Design review of the part built by this model. Coordinates are the model's own, in mm. A direction names the side the tool comes from. Coordinates: 2 decimals unless noted, no trailing zeros. Order: outer loops, then holes, each group sorted by start corner. A loop starts at its lowest first (then second) coordinate and runs counter-clockwise, first axis right, second up. Notation, with made-up numbers: M -19,51 L 19,51 A30 cw 19,77 Z; hole C 87,49.25 d8. An arc over 180 degrees is marked long. Answer as a JSON object with one key per item and string values.
from build123d import *

# Parameters (mm, degrees)
SKETCH001_R          = 2.5
PAD_DEPTH            = 7.5
PAD_DEPTH_BACK       = 1.5
SKETCH_R             = 1.75
SKETCH_R_2           = 2.5
PAD001_DEPTH         = 6
SKETCH003_W          = 20
SKETCH003_H          = 3
POCKET_DEPTH         = 100
POCKET_DEPTH_BACK    = -100
FILLET_R             = 5
FILLET001_R          = 2
FILLET002_R          = 1
SKETCH004_R          = 4.25
POCKET001_DEPTH      = 2
POCKET001_DEPTH_BACK = -2
SKETCH005_R          = 5.5
POCKET002_DEPTH      = 5
SKETCH006_R          = 2.25
POCKET003_DEPTH      = 4


with BuildPart() as part:
    # Sketch001 → Pad (new body, two sides)
    with BuildSketch(Plane.XY) as pad_sk:
        Polygon((74, -6), (74, 0), (0, 0), (0, -6), (6.75, -6), (6.75, -20.25), (17.25, -20.25), (17.25, -6), (46.75, -6), (46.75, -20.25), (57.25, -20.25), (57.25, -6), align=None)
        with Locations((12, -15)):
            Circle(SKETCH001_R, mode=Mode.SUBTRACT)
        with Locations((52, -15)):
            Circle(SKETCH001_R, mode=Mode.SUBTRACT)
    extrude(amount=PAD_DEPTH)
    extrude(pad_sk.sketch, amount=-PAD_DEPTH_BACK)

    # Sketch → Pad001 (join)
    with BuildSketch(Plane.XZ):
        with BuildLine():
            ThreePointArc((37.87, 12.75), (34.37, 16.25), (30.87, 12.75))
            Line((30.87, 12.75), (30.87, 4.75))
            ThreePointArc((30.87, 4.75), (34.37, 1.25), (37.87, 4.75))
            Line((37.87, 12.75), (37.87, 4.75))
        make_face()
        with Locations((34.37, 12.75)):
            Circle(SKETCH_R, mode=Mode.SUBTRACT)
        with BuildLine():
            ThreePointArc((52.8, 12.75), (48.3, 17.25), (43.8, 12.75))
            Line((43.8, 12.75), (43.8, 4.75))
            ThreePointArc((43.8, 4.75), (48.3, 0.25), (52.8, 4.75))
            Line((52.8, 12.75), (52.8, 4.75))
        make_face()
        with Locations((48.3, 12.75)):
            Circle(SKETCH_R_2, mode=Mode.SUBTRACT)
        with BuildLine():
            ThreePointArc((69.87, 12.75), (66.37, 16.25), (62.87, 12.75))
            Line((62.87, 12.75), (62.87, 4.75))
            ThreePointArc((62.87, 4.75), (66.37, 1.25), (69.87, 4.75))
            Line((69.87, 12.75), (69.87, 4.75))
        make_face()
        with Locations((66.37, 12.75)):
            Circle(SKETCH_R, mode=Mode.SUBTRACT)
    extrude(amount=PAD001_DEPTH)

    # Sketch003 → Pocket (cut, two sides)
    with BuildSketch(Plane.YZ) as pocket_sk:
        with Locations((-12.2, 3)):
            Rectangle(SKETCH003_W, SKETCH003_H)
    extrude(amount=-POCKET_DEPTH, mode=Mode.SUBTRACT)
    extrude(pocket_sk.sketch, amount=-POCKET_DEPTH_BACK, mode=Mode.SUBTRACT)

    # Fillet
    fillet_edges = [part.edges().sort_by_distance(p)[0] for p in [
        (46.75, -20.25, 0),
        (46.75, -20.25, 6),
        (57.25, -20.25, 6),
        (57.25, -20.25, 0),
        (17.25, -20.25, 0),
        (17.25, -20.25, 6),
        (6.75, -20.25, 6),
        (6.75, -20.25, 0),
    ]]
    fillet(fillet_edges, radius=FILLET_R)

    # Fillet001
    fillet001_edges = [part.edges().sort_by_distance(p)[0] for p in [
        (74, 0, 3),
        (0, 0, 3),
    ]]
    fillet(fillet001_edges, radius=FILLET001_R)

    # Fillet002
    fillet002_edges = [part.edges().sort_by_distance(p)[0] for p in [
        (49.775, -6, 7.5),
        (52.8, -3, 7.5),
        (46.75, -6, 6),
        (57.25, -6, 6),
        (62.87, -3, 7.5),
        (69.87, -3, 7.5),
        (57.25, -6, 0),
        (46.75, -6, 0),
        (6.75, -6, 6),
        (6.75, -6, 0),
        (43.8, -3, 7.5),
        (30.87, -3, 7.5),
        (37.87, -3, 7.5),
        (17.25, -6, 6),
        (17.25, -6, 0),
    ]]
    fillet(fillet002_edges, radius=FILLET002_R)

    # Sketch004 → Pocket001 (cut, two sides)
    with BuildSketch(Plane.XY) as pocket001_sk:
        with Locations((12, -15)):
            Circle(SKETCH004_R)
        with Locations((52, -15)):
            Circle(SKETCH004_R)
    extrude(amount=-POCKET001_DEPTH, mode=Mode.SUBTRACT)
    extrude(pocket001_sk.sketch, amount=-POCKET001_DEPTH_BACK, mode=Mode.SUBTRACT)

    # Sketch005 → Pocket002 (cut)
    with BuildSketch(Plane.XY.offset(6.9)):
        with Locations((12, -15)):
            Circle(SKETCH005_R)
        with Locations((52, -15)):
            Circle(SKETCH005_R)
    extrude(amount=POCKET002_DEPTH, mode=Mode.SUBTRACT)

    # Sketch006 → Pocket003 (cut)
    with BuildSketch(Plane.XZ):
        with Locations((34.37, 12.75)):
            Circle(SKETCH006_R)
        with Locations((66.37, 12.75)):
            Circle(SKETCH006_R)
    extrude(amount=POCKET003_DEPTH, mode=Mode.SUBTRACT)


solid = part.part
1) Tool access review of faces 4 (the cylindrical face through (52.1, -9.5, 7.2)), 5 (the flat face through (46.75, -11, 0)), 6 (the cylindrical face through (48.63, -17.59, 0.02)): name each direction out of +Z, -Z, +X, -X, +Y, -Y from which nothing blocks a thin tool from reaching the whole face with its end or side.
Taken from the geometry:
{"face 4": "+Z, -Y", "face 5": "+Z, -Z, -Y", "face 6": "-Z"}
2) Mouldability with a two-part tool opening along Z and no side actions: class faces 1 (the flat face through (36, -3, -1.5)), 2 (the flat face through (36, -2.2, 3)), 3 (the flat face through (57.25, -11, 0)) as released by +Z, released by -Z, zero draft, split by the parting line, or undercut.
Taken from the geometry:
{"face 1": "released by -Z", "face 2": "undercut", "face 3": "zero draft"}
3) Add section C-C (x = 8.5). State the section outline as (y, z) points.
Taken from the geometry:
{"outline": "M -19.05,-1.5 L -17.41,-1.5 L -17.41,1.5 L -19.05,1.5 Z; M -19.05,4.5 L -2.2,4.5 L -2.2,1.5 L -12.59,1.5 L -12.59,-1.5 L 0,-1.5 L 0,7.5 L -10.76,7.5 L -10.76,6.9 L -19.05,6.9 Z"}
4) Add section A-A (x = 34.37). State the section outline as (y, z) points.
Taken from the geometry:
{"outline": "M -6,-1.5 L 0,-1.5 L 0,10.5 L -4,10.5 L -4,11 L -6,11 L -6,4.5 L -2.2,4.5 L -2.2,1.5 L -6,1.5 Z; M -6,14.5 L -4,14.5 L -4,15 L 0,15 L 0,16.25 L -6,16.25 Z"}
5) Insertion check: pin 1 Ø2 at (y, z) = (-4, 10.5) entering from +X; pin 2 Ø0.9 at (y, z) = (-11, 0.5) entering from -X; pin 3 Ø8 at (x, y) = (12, -15) entering from +Z; pin 4 Ø11 at (x, y) = (12, -15) entering from -Z. Each pin has a flat end and moves straight along its axis. Give the tip position at first contact, or say it passes through.
Taken from the geometry:
{"pin 1": "stops at x = 69.87", "pin 2": "stops at x = 6.75", "pin 3": "stops at z = 6.9", "pin 4": "stops at z = -1.5"}
6) Add section B-B (y = -8.75). State the section outline as (x, z) points, and give its area (3 significant figures).
Taken from the geometry:
{"outline": "M 6.75,-1.5 L 17.25,-1.5 L 17.25,1.5 L 6.75,1.5 Z; M 6.75,4.5 L 17.25,4.5 L 17.25,7.5 L 6.75,7.5 Z; M 46.75,-1.5 L 57.25,-1.5 L 57.25,1.5 L 46.75,1.5 Z; M 46.75,4.5 L 57.25,4.5 L 57.25,7.5 L 46.75,7.5 Z", "area": "126 mm2"}
7) To check wall thickness, follow L1, parallel to X at y = -15, z = 5.8; L2, parallel to Z at x = 34.37, y = -4.5; L3, parallel to Y at x = 52, z = 5.6. State the ranges of each line that lie inside material, in increasing order.
Taken from the geometry:
{"L1": "x = 6.75 to 9.5, 14.5 to 17.25, 46.75 to 49.5, 54.5 to 57.25", "L2": "z = -1.5 to 1.5, 4.5 to 11, 14.5 to 16.25", "L3": "y = -20.25 to -17.5, -12.5 to 0"}
